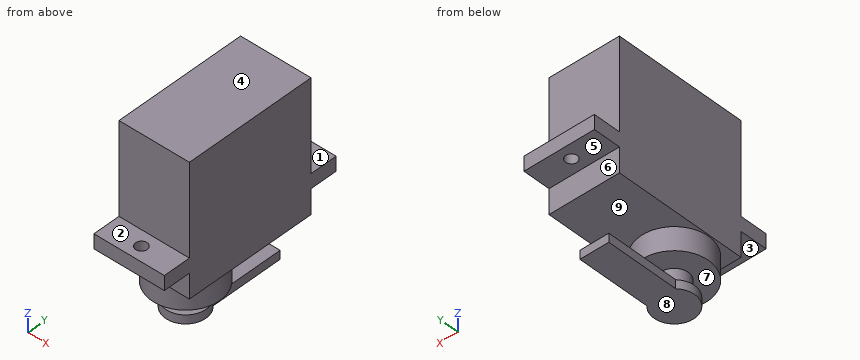
from build123d import *

# Parameters (mm, degrees)
CROQUIS1_W              = 12.2
CROQUIS1_H              = 22.8
SALIENTE_EXTRUIR1_DEPTH = 22.7
CROQUIS2_W              = 12.2
CROQUIS2_H              = 32.2
SALIENTE_EXTRUIR2_DEPTH = 2.5
CROQUIS3_R              = 1
CORTAR_EXTRUIR1_DEPTH   = 4.5
CROQUIS4_R              = 5.9
SALIENTE_EXTRUIR3_DEPTH = 4
CROQUIS5_R              = 2.4
SALIENTE_EXTRUIR4_DEPTH = 2.8
CROQUIS6_R              = 3.5
SALIENTE_EXTRUIR5_DEPTH = 1.5
CROQUIS7_W              = 5
CROQUIS7_H              = 13
SALIENTE_EXTRUIR6_DEPTH = 1.5


with BuildPart() as part:
    # Croquis1 → Saliente-Extruir1 (new body)
    with BuildSketch(Plane.XY.offset(-4.3)):
        with Locations((0, 5.5)):
            Rectangle(CROQUIS1_W, CROQUIS1_H)
    extrude(amount=SALIENTE_EXTRUIR1_DEPTH)

    # Croquis2 → Saliente-Extruir2 (add)
    with BuildSketch(Plane.XY):
        with Locations((0, 5.5)):
            Rectangle(CROQUIS2_W, CROQUIS2_H)
    extrude(amount=SALIENTE_EXTRUIR2_DEPTH)

    # Croquis3 → Cortar-Extruir1 (cut)
    with BuildSketch(Plane.XY.offset(-1)):
        with Locations((0, -8.3)):
            Circle(CROQUIS3_R)
        with Locations((0, 19.3)):
            Circle(CROQUIS3_R)
    extrude(amount=CORTAR_EXTRUIR1_DEPTH, mode=Mode.SUBTRACT)

    # Croquis4 → Saliente-Extruir3 (add)
    with BuildSketch(Plane.XY.offset(-8.3)):
        with Locations(Location((0, 0, 0), (0, 0, 270))):
            Circle(CROQUIS4_R)
    extrude(amount=SALIENTE_EXTRUIR3_DEPTH)

    # Croquis5 → Saliente-Extruir4 (add)
    with BuildSketch(Plane.XY.offset(-11.1)):
        Circle(CROQUIS5_R)
    extrude(amount=SALIENTE_EXTRUIR4_DEPTH)

    # Croquis6 → Saliente-Extruir5 (add)
    with BuildSketch(Plane.XY.offset(-12.6)):
        Circle(CROQUIS6_R)
    extrude(amount=SALIENTE_EXTRUIR5_DEPTH)

    # Croquis7 → Saliente-Extruir6 (add)
    with BuildSketch(Plane.XY.offset(-12.6)):
        with Locations((0, 8.5)):
            Rectangle(CROQUIS7_W, CROQUIS7_H)
    extrude(amount=SALIENTE_EXTRUIR6_DEPTH)


solid = part.part
For this review, take the finished solid that the model builds, in its own axes (mm). Face numbers are marked on the shaded views. A direction names the side the tool comes from. Round coordinates to 2 decimals unless told otherwise and drop trailing zeros. Write each loop counter-clockwise with the first axis right and the second up, starting at its lowest first coordinate (ties: lowest second). Pieces come first, ordered by that corner, then holes. Notation, with made-up numbers: (-17.75, 64.5) - (-10.75, 64.5) arc R26 cw to (-10.75, 100.5) - close; hole circle Ø5 at (32.25, 15.25). An arc over 180 degrees is marked (long way). Use a Markdown table: item, result.
Q1. We need section B-B (z = 0.5). Give the boundary of the cut face in (x, y).
Derived:
| item | result |
|---|---|
| outline | (-6.1, -10.6) - (6.1, -10.6) - (6.1, 21.6) - (-6.1, 21.6) - close; hole circle Ø2 at (0, -8.3); hole circle Ø2 at (0, 19.3) |
Q2. We need section A-A (y = 8). Give the boundary of the cut face in (x, z).
Derived:
| item | result |
|---|---|
| outline | (-6.1, -4.3) - (6.1, -4.3) - (6.1, 18.4) - (-6.1, 18.4) - close; (-2.5, -12.6) - (2.5, -12.6) - (2.5, -11.1) - (-2.5, -11.1) - close |
Q3. Clearance check with flat-ended pins moving along their axes: pin 1 (1.2 mm diameter, centred on x = 0, y = -8.3, fed in from -Z); pin 2 (1.4 mm diameter, centred on x = -2, y = 20, fed in from +Z); pin 3 (2.5 mm diameter, centred on x = 2, y = 18.5, fed in from -Z); pin 4 (1.2 mm diameter, centred on y = 11.5, z = -11.5, fed in from -X). State where each tip first meets the part, or that it passes through.
Derived:
| item | result |
|---|---|
| pin 1 | passes through |
| pin 2 | stops at z = 2.5 |
| pin 3 | stops at z = 0 |
| pin 4 | stops at x = -2.5 |
Q4. We need section C-C (x = -3). Give the boundary of the cut face in (y, z).
Derived:
| item | result |
|---|---|
| outline | (-10.6, 0) - (-5.9, 0) - (-5.9, -4.3) - (-5.08, -4.3) - (-5.08, -8.3) - (5.08, -8.3) - (5.08, -4.3) - (16.9, -4.3) - (16.9, 0) - (21.6, 0) - (21.6, 2.5) - (16.9, 2.5) - (16.9, 18.4) - (-5.9, 18.4) - (-5.9, 2.5) - (-10.6, 2.5) - close; (-1.8, -12.6) - (1.8, -12.6) - (1.8, -11.1) - (-1.8, -11.1) - close |
Q5. The part is to be moulded in two halves that separate along Z. For the marked faces 6, 7, 8 and 9, say which applies: pulls with the +Z half, pulls with the -Z half, needs draft (parallel to the pull), parting line crosses it, or undercut.
Derived:
| item | result |
|---|---|
| face 6 | needs draft |
| face 7 | undercut |
| face 8 | pulls with the -Z half |
| face 9 | undercut |
Q6. Machinability: for the marked faces 1, 2, 3, 4 and 5, which of the approach directions +Z, -Z, +X, -X, +Y, -Y give a long, thin tool a straight path to every point of the face, cutting with its end or side? Answer none if there is none.
Derived:
| item | result |
|---|---|
| face 1 | +Z, +X, -X, +Y |
| face 2 | +Z, +X, -X, -Y |
| face 3 | -Z, +X, -X, -Y |
| face 4 | +Z, +X, -X, +Y, -Y |
| face 5 | -Z, +X, -X, +Y |
Q7. Wall thickness on line 1 along Y through (x, z) = (0, 1.3); line 2 along Z through (x, y) = (-1.5, 9.5); line 3 along X through (y, z) = (-8.3, 0.75): over which ranges is each line inside the solid? List them lowest first.
Derived:
| item | result |
|---|---|
| line 1 | y = -10.6 to -9.3, -7.3 to 18.3, 20.3 to 21.6 |
| line 2 | z = -12.6 to -11.1, -4.3 to 18.4 |
| line 3 | x = -6.1 to -1, 1 to 6.1 |
Q8. We need section D-D (y = 19.3). Give the boundary of the cut face in (x, z), plus the area to 3 significant figures.
Derived:
| item | result |
|---|---|
| outline | (-6.1, 0) - (-1, 0) - (-1, 2.5) - (-6.1, 2.5) - close; (1, 0) - (6.1, 0) - (6.1, 2.5) - (1, 2.5) - close |
| area | 25.5 mm2 |
